from build123d import *

# Parameters (mm, degrees)
SKETCH_1_W          = 10
SKETCH_1_H          = 20
SKETCH_1_W_2        = 7.6
SKETCH_1_H_2        = 17.6
EXTRUDE_1_DEPTH     = 680
SKETCH_2_R          = 2
CUT_EXTRUDE_1_DEPTH = 681.312428227


with BuildPart() as part:
    # ｽｹｯﾁ1 → 押し出し-薄板1 (new body)
    with BuildSketch(Plane.XY):
        Rectangle(SKETCH_1_W, SKETCH_1_H)
        Rectangle(SKETCH_1_W_2, SKETCH_1_H_2, mode=Mode.SUBTRACT)
    extrude(amount=EXTRUDE_1_DEPTH)

    # ｽｹｯﾁ2 → ｶｯﾄ - 押し出し1 (cut, through all)
    with BuildSketch(Plane(origin=(0, 10, 0), x_dir=(1, 0, 0), z_dir=(0, 1, 0))):
        with Locations(Location((0, -665, 0), (0, 0, 270))):
            Circle(SKETCH_2_R)
        with Locations(Location((0, -675, 0), (0, 0, 270))):
            Circle(SKETCH_2_R)
        with Locations(Location((0, -5, 0), (0, 0, 270))):
            Circle(SKETCH_2_R)
        with Locations(Location((0, -15, 0), (0, 0, 270))):
            Circle(SKETCH_2_R)
        with Locations(Location((0, -525, 0), (0, 0, 270))):
            Circle(SKETCH_2_R)
        with Locations(Location((0, -405, 0), (0, 0, 270))):
            Circle(SKETCH_2_R)
        with Locations(Location((0, -215, 0), (0, 0, 270))):
            Circle(SKETCH_2_R)
        with Locations(Location((0, -385, 0), (0, 0, 270))):
            Circle(SKETCH_2_R)
    extrude(amount=-CUT_EXTRUDE_1_DEPTH, mode=Mode.SUBTRACT)


solid = part.part
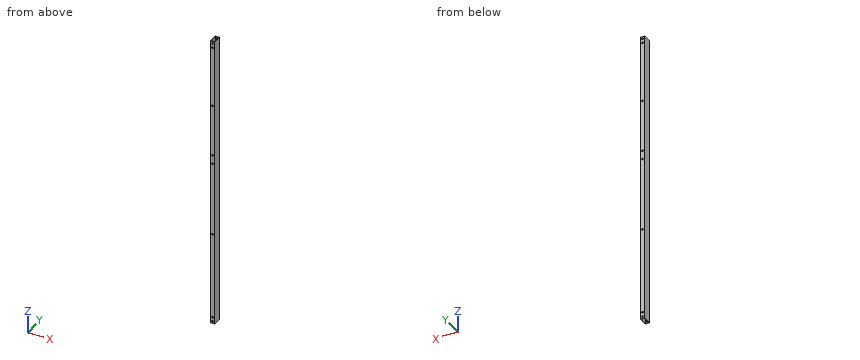
Geometry check sheet. Reference: the model listing, model coordinates, mm. Give positions to 0.01 mm unless a question says otherwise; leave off trailing zeros. Order: outer loops, then holes, each group sorted by start corner. A loop starts at its lowest first (then second) coordinate and runs counter-clockwise, first axis right, second up. Notation, with made-up numbers: M 31,62 L 51,62 A8 cw 51,74 Z; hole C -8.75,11 d3. An arc over 180 degrees is marked long. Use a Markdown table: item, result.
Item 1: Section check A-A (y = 2). Record the cut outline in (x, z), and give its area (3 significant figures).
Answers follow:
| item | result |
|---|---|
| outline | M -5,0 L -3.8,0 L -3.8,680 L -5,680 Z; M 3.8,0 L 5,0 L 5,680 L 3.8,680 Z |
| area | 1,630 mm2 |
Item 2: Material ranges on line 1 along Y through (x, z) = (2.25, 403); line 2 along X through (y, z) = (8.5, 175.5); line 3 along X through (y, z) = (9.3, 525), recorded low to high.
Answers follow:
| item | result |
|---|---|
| line 1 | y = -10 to -8.8, 8.8 to 10 |
| line 2 | x = -5 to -3.8, 3.8 to 5 |
| line 3 | x = -5 to -2, 2 to 5 |
Item 3: Depth check by flat-ended pin: P1, Ø2.5, axis at x = 0, z = 525, coming from the -Y side; P2, Ø5, axis at x = 0, z = 5, coming from the -Y side. Enter the tip coordinate at first touch or a pass-through.
Answers follow:
| item | result |
|---|---|
| P1 | passes through |
| P2 | stops at y = -10 |
Item 4: Section check B-B (z = 86). Record the cut outline in (x, y).
Answers follow:
| item | result |
|---|---|
| outline | M -5,-10 L 5,-10 L 5,10 L -5,10 Z; hole M -3.8,-8.8 L 3.8,-8.8 L 3.8,8.8 L -3.8,8.8 Z |
